The listing builds one solid part. Answer for the finished solid, in the listing's coordinates (mm). Coordinates: 2 decimals unless noted, no trailing zeros. Order: outer loops, then holes, each group sorted by start corner. A loop starts at its lowest first (then second) coordinate and runs counter-clockwise, first axis right, second up. Notation, with made-up numbers: (44, 61) -> (72, 61) arc R12 ccw to (72, 83) -> close; hole circle Ø1 at (-11, 24). An arc over 180 degrees is marked (long way). Return JSON: item names as keys, results as strings.
```python
from build123d import *

# Parameters (mm, degrees)
BOSS_EXTRUDE1_DEPTH      = 812.8
BOSS_EXTRUDE1_DEPTH_BACK = 812.8
CUT_EXTRUDE1_DEPTH       = 814.295942447


with BuildPart() as part:
    # Sketch4 → Boss-Extrude1 (new, two sides: drawn at the far end of the back side and taken through both)
    with BuildSketch(Plane(origin=(0, 0, 0), x_dir=(0, 0, -1), z_dir=(1, 0, 0)).offset(-BOSS_EXTRUDE1_DEPTH_BACK)):
        with BuildLine():
            Line((12.7, -11.43), (12.7, 11.43))
            ThreePointArc((12.7, 11.43), (12.328025612, 12.328025612), (11.43, 12.7))
            Line((11.43, 12.7), (-11.43, 12.7))
            ThreePointArc((-11.43, 12.7), (-12.328025612, 12.328025612), (-12.7, 11.43))
            Line((-12.7, 11.43), (-12.7, -11.43))
            ThreePointArc((-12.7, -11.43), (-12.328025612, -12.328025612), (-11.43, -12.7))
            Line((-11.43, -12.7), (11.43, -12.7))
            ThreePointArc((11.43, -12.7), (12.328025612, -12.328025612), (12.7, -11.43))
        make_face()
        with BuildLine():
            Line((11.049, 9.9441), (11.049, -9.9441))
            ThreePointArc((11.049, -9.9441), (10.725382283, -10.725382283), (9.9441, -11.049))
            Line((9.9441, -11.049), (-9.9441, -11.049))
            ThreePointArc((-9.9441, -11.049), (-10.725382283, -10.725382283), (-11.049, -9.9441))
            Line((-11.049, -9.9441), (-11.049, 9.9441))
            ThreePointArc((-11.049, 9.9441), (-10.725382283, 10.725382283), (-9.9441, 11.049))
            Line((-9.9441, 11.049), (9.9441, 11.049))
            ThreePointArc((9.9441, 11.049), (10.725382283, 10.725382283), (11.049, 9.9441))
        make_face(mode=Mode.SUBTRACT)
    extrude(amount=BOSS_EXTRUDE1_DEPTH + BOSS_EXTRUDE1_DEPTH_BACK)

    # Sketch5 → Cut-Extrude1 (cut, through all)
    with BuildSketch(Plane.XY.offset(12.7)):
        Polygon((812.8, -12.7), (807.168955569, 12.7), (812.8, 12.7), align=None)
    cut_extrude1 = extrude(amount=-CUT_EXTRUDE1_DEPTH, mode=Mode.SUBTRACT)

    # Mirror1: Cut-Extrude1 across plane
    add(cut_extrude1.mirror(Plane(origin=(0, 0, 0), x_dir=(0, 0, 1), z_dir=(1, 0, 0))), mode=Mode.SUBTRACT)


solid = part.part
```
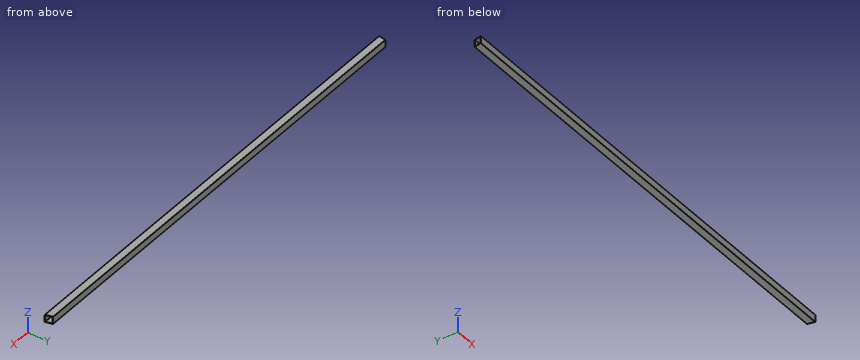
Item 1: A flat-ended cylindrical pin translates along its axis: pin 1 (1 mm diameter, centred on y = 1, z = 9.5, fed in from +X) (3 decimals). Find the tip coordinate at first contact, or state that the pin passes through.
Answer list:
{"pin 1": "through"}
Item 2: The part is cut by section C-C on y = -4.75. Determine the outline of the cut face in (x, z), plus the area to 3 significant figures.
Answer list:
{"outline": "(-811.04, -12.7) -> (811.04, -12.7) -> (811.04, -11.05) -> (-811.04, -11.05) -> close; (-811.04, 11.05) -> (811.04, 11.05) -> (811.04, 12.7) -> (-811.04, 12.7) -> close", "area": "5,360 mm2"}
Item 3: The part is cut by section B-B on x = 334. Determine the outline of the cut face in (y, z), plus the area to 3 significant figures.
Answer list:
{"outline": "(-12.7, -11.43) arc R1.27 ccw to (-11.43, -12.7) -> (11.43, -12.7) arc R1.27 ccw to (12.7, -11.43) -> (12.7, 11.43) arc R1.27 ccw to (11.43, 12.7) -> (-11.43, 12.7) arc R1.27 ccw to (-12.7, 11.43) -> close; hole (-11.05, -9.94) arc R1.1 ccw to (-9.94, -11.05) -> (9.94, -11.05) arc R1.1 ccw to (11.05, -9.94) -> (11.05, 9.94) arc R1.1 ccw to (9.94, 11.05) -> (-9.94, 11.05) arc R1.1 ccw to (-11.05, 9.94) -> close", "area": "157 mm2"}
Item 4: The part is cut by section A-A on z = 0.5. Determine the outline of the cut face in (x, y).
Answer list:
{"outline": "(-812.8, -12.7) -> (812.8, -12.7) -> (812.43, -11.05) -> (-812.43, -11.05) -> close; (-807.53, 11.05) -> (807.53, 11.05) -> (807.17, 12.7) -> (-807.17, 12.7) -> close"}
Item 5: Find the intervals of material crossed by probe 1 along Y at (x, z) = (-477, -1); probe 2 along Y at (x, z) = (-558, 11.75), in increasing order.
Answer list:
{"probe 1": "-12.7 to -11.05, 11.05 to 12.7", "probe 2": "-12.66 to 12.66"}
